Study the drawing (mm; zero at the part's minimum x, y, z) and answer. Coordinates: 2 decimals unless noted, no trailing zeros. Write each loop counter-clockwise with the first axis right and the second up, starting at its lowest first coordinate (ties: lowest second). Pieces come first, ordered by that corner, then holes. Notation, with made-up numbers: (66.5, 0) -> (82.5, 0) arc R19 ccw to (82.5, 7) -> close; hole circle Ø6 at (39, 49.5). An arc over 180 degrees is marked (long way). Write item = value, one per line. Start each with the question number.
1) Section C-C (x = 13.5) is taken. Determine the outline of the cut face in (y, z), plus the area to 3 significant figures.
2) Section B-B (z = 49) is taken. Determine the outline of the cut face in (x, y).
3) Flat-ended cylindrical pins translate along their axes: pin 1 Ø5 at (y, z) = (36, 36) entering from -X; pin 2 Ø10 at (y, z) = (32.5, 10) entering from +X; pin 3 Ø1.5 at (y, z) = (68, 9) entering from -X. Find the tip coordinate at first contact, or state that the pin passes through.
4) Section A-A (y = 58) is taken. Determine the outline of the cut face in (x, z), plus the area to 3 significant figures.
5) Find the intervals of material crossed by line 1 along X through (y, z) = (31.5, 43); line 2 along X through (y, z) = (45.5, 17) (3 decimals); line 3 along Z through (x, y) = (4, 25), in increasing order. Write a range as from..to.
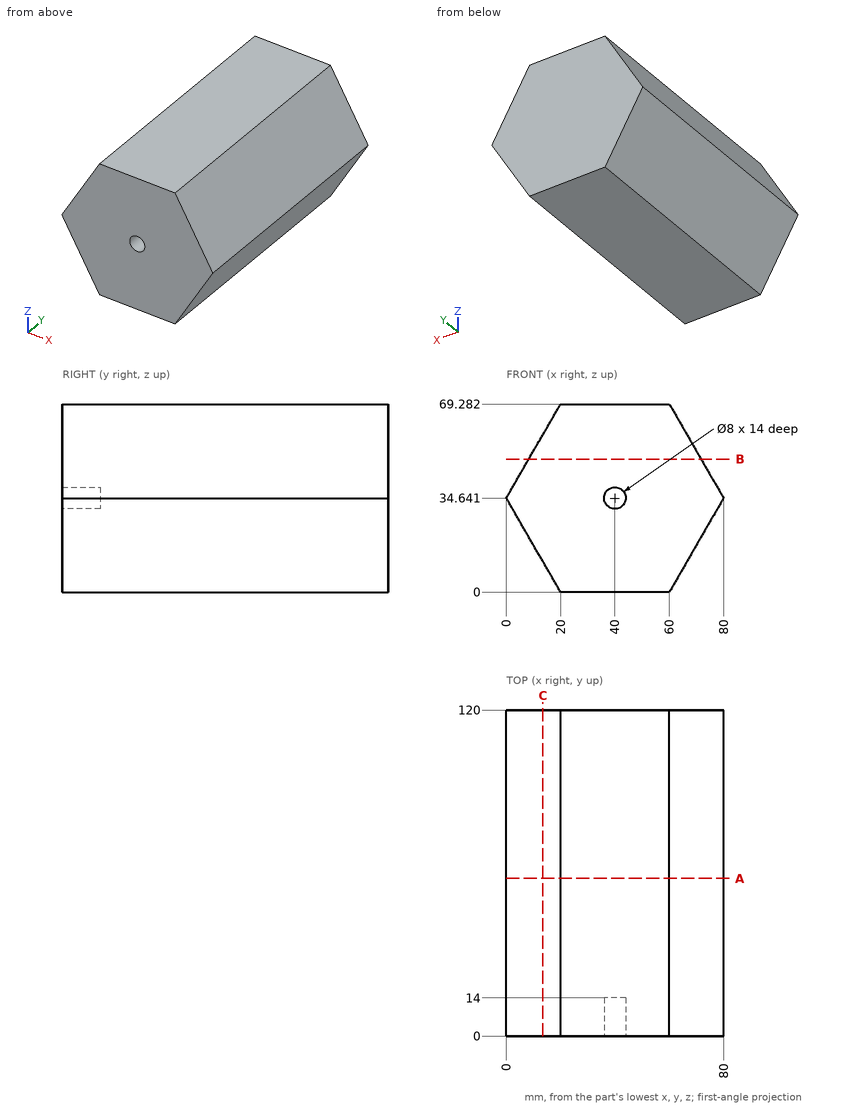
Answer key:
q1.outline = (0, 11.26) -> (120, 11.26) -> (120, 58.02) -> (0, 58.02) -> close
q1.area = 5,610 mm^2
q2.outline = (8.29, 0) -> (71.71, 0) -> (71.71, 120) -> (8.29, 120) -> close
q3.pin_1 = 0
q3.pin_2 = 68.66
q3.pin_3 = 14.37
q4.outline = (0, 34.64) -> (20, 0) -> (60, 0) -> (80, 34.64) -> (60, 69.28) -> (20, 69.28) -> close
q4.area = 4,160 mm^2
q5.line_1 = 4.83..75.17
q5.line_2 = 10.185..69.815
q5.line_3 = 27.71..41.57
